Geometry: final body of the model. Coordinates: model frame, mm. Face numbers are marked on the shaded views. Give positions to 0.01 mm unless a question says otherwise; leave off trailing zeros. Write each loop counter-clockwise with the first axis right and the second up, starting at its lowest first coordinate (ties: lowest second). Pieces come first, ordered by that corner, then holes.
```python
from build123d import *

# Parameters (mm, degrees)
F0_R           = 4.825
F1_DEPTH       = 33
F3_DEPTH       = 6.5
F4_R           = 0.2
F8_DEPTH       = 5
F9_R           = 1.05
F10_DEPTH      = 4.8260001
F10_DEPTH_BACK = 4.8260001
F12_START      = 3.325
F12_DEPTH      = 1.5010001
F14_START      = -3.325
F13_R          = 2
F14_DEPTH      = 1.5010001118


with BuildPart() as f1:
    # F0 (on Top) → F1 (new body)
    with BuildSketch(Plane.XY):
        Circle(F0_R)
    extrude(amount=F1_DEPTH)

    # F2 (on Front) → F3 (join)
    with BuildSketch(Plane.XZ):
        with BuildLine():
            ThreePointArc((-1.5, 3.5), (0, 2), (1.5, 3.5))
            Line((1.5, 3.5), (1.5, 6.5))
            ThreePointArc((1.5, 6.5), (0, 8), (-1.5, 6.5))
            Line((-1.5, 6.5), (-1.5, 3.5))
        make_face()
    extrude(amount=F3_DEPTH)

    # F4
    f4_edges = [f1.edges().sort_by_distance(p)[0] for p in [
        (0, -6.5, 2),
        (1.5, -6.5, 5),
        (0, -6.5, 8),
        (-1.5, -6.5, 5),
    ]]
    fillet(f4_edges, radius=F4_R)

    # F5 (on Front) → F6 (revolve)
    with BuildSketch(Plane.XZ):
        with BuildLine():
            Line((0, 0), (-4.825, 0))
            ThreePointArc((-4.825, 0), (-2.5263919431, -1.1163524169), (0, -1.5))
            Line((0, -1.5), (0, 0))
        make_face()
    revolve(axis=Axis((0, 0, -1.4078605181), (0, 0, -1)))

    # F7 (on face) → F8 (cut)
    with BuildSketch(Plane.XY.offset(33)):
        with BuildLine():
            ThreePointArc((1.5, 4.585915939), (0, 4.825), (-1.5, 4.585915939))
            Line((-1.5, 4.585915939), (-1.5, -4.585915939))
            ThreePointArc((-1.5, -4.585915939), (0, -4.825), (1.5, -4.585915939))
            Line((1.5, -4.585915939), (1.5, 4.585915939))
        make_face()
    extrude(amount=-F8_DEPTH, mode=Mode.SUBTRACT)

    # F9 (on Right) → F10 (cut, two sides)
    with BuildSketch(Plane.YZ) as f10_sk:
        with Locations((0, 30.5)):
            Circle(F9_R)
    extrude(amount=F10_DEPTH, mode=Mode.SUBTRACT)
    extrude(f10_sk.sketch, amount=-F10_DEPTH_BACK, mode=Mode.SUBTRACT)

    # F11 (on Right) → F12 (cut)
    with BuildSketch(Plane.YZ.offset(F12_START)):
        Polygon((1.1835680518, 28.45), (2.3671361037, 30.5), (1.1835680518, 32.55), (-1.1835680518, 32.55), (-2.3671361037, 30.5), (-1.1835680518, 28.45), align=None)
    extrude(amount=F12_DEPTH, mode=Mode.SUBTRACT)

    # F13 (on Right) → F14 (cut)
    with BuildSketch(Plane.YZ.offset(F14_START)):
        with Locations((0, 30.5)):
            Circle(F13_R)
    extrude(amount=-F14_DEPTH, mode=Mode.SUBTRACT)


solid = f1.part
```
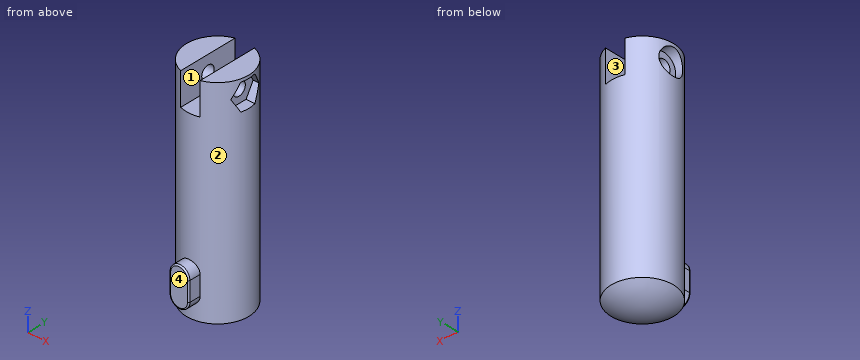
Item 1: Line query: L1, parallel to X at y = -1.5, z = 7.5; L2, parallel to Y at x = -3.5, z = 6; L3, parallel to Z at x = 1.95, y = 0. Output: solid intervals per line, ascending.
Found:
L1: x = -4.59 to 4.59
L2: y = -3.32 to 3.32
L3: z = -1.27 to 29.45, 31.55 to 33
Item 2: Section C-C, the plane x = -3.75. Return the cut outline in (y, z), plus the area to 3 significant figures.
Found:
outline: (-3.04, 0) arc R7.64 ccw to (3.04, 0) - (3.04, 33) - (-3.04, 33) - close; hole circle Ø4 at (0, 30.5)
area: 190 mm2
Item 3: Pin query (flat end, axial travel): pin 1 Ø3 at (y, z) = (0, 30.5) entering from -X (3 decimals); pin 2 Ø1 at (y, z) = (-4.5, 29.5) entering from -X; pin 3 Ø1.4 at (y, z) = (-5, 5) entering from -X. Return the tip coordinate at first contact, or that it passes through.
Found:
pin 1: stops at x = -3.325
pin 2: stops at x = -2.7
pin 3: stops at x = -2.19
Item 4: Section D-D, the plane y = 3.5. Return the cut outline in (x, z), plus the area to 3 significant figures.
Found:
outline: (-3.32, 0) arc R7.76 ccw to (3.32, 0) - (3.32, 33) - (1.5, 33) - (1.5, 28) - (-1.5, 28) - (-1.5, 33) - (-3.32, 33) - close
area: 208 mm2
Item 5: Section A-A, the plane y = 0. Return the cut outline in (x, z) (3 decimals).
Found:
outline: (-4.825, 0) arc R8.51 ccw to (4.825, 0) - (4.825, 28.45) - (3.325, 28.45) - (3.325, 29.45) - (1.5, 29.45) - (1.5, 28) - (-1.5, 28) - (-1.5, 29.45) - (-3.325, 29.45) - (-3.325, 28.5) - (-4.825, 28.5) - close; (-4.825, 32.5) - (-3.325, 32.5) - (-3.325, 31.55) - (-1.5, 31.55) - (-1.5, 33) - (-4.825, 33) - close; (1.5, 31.55) - (3.325, 31.55) - (3.325, 32.55) - (4.825, 32.55) - (4.825, 33) - (1.5, 33) - close
Item 6: Section B-B, the plane x = 0. Return the cut outline in (y, z) (3 decimals), plus the area to 3 significant figures.
Found:
outline: (-6.5, 2.2) arc R0.2 ccw to (-6.3, 2) - (-4.825, 2) - (-4.825, 0) arc R8.51 ccw to (4.825, 0) - (4.825, 28) - (-4.825, 28) - (-4.825, 8) - (-6.3, 8) arc R0.2 ccw to (-6.5, 7.8) - close
area: 290 mm2
Item 7: Pull-direction query (X, two-part tool) for the marked faces 1, 2, 3 and 4; classes: +X half, -X half, draft (parallel to the pull), parting line (faces both ways), or undercut.
Found:
face 1: undercut
face 2: parting line
face 3: undercut
face 4: draft
